from build123d import *

# Parameters (mm, degrees)
SKETCH1_R           = 48.895
SKETCH1_R_2         = 45.72
BOSS_EXTRUDE1_DEPTH = 6.35
SKETCH2_R           = 48.895
SKETCH2_R_2         = 12.7
BOSS_EXTRUDE2_DEPTH = 3.175
SKETCH3_R           = 3.175
BOSS_EXTRUDE3_DEPTH = 46.825


with BuildPart() as part:
    # Sketch1 → Boss-Extrude1 (new body)
    with BuildSketch(Plane(origin=(0, 0, 0), x_dir=(1, 0, 0), z_dir=(0, 1, 0))):
        with Locations(Location((0, 0, 0), (0, 0, 270))):
            Circle(SKETCH1_R)
        with Locations(Location((0, 0, 0), (0, 0, 270))):
            Circle(SKETCH1_R_2, mode=Mode.SUBTRACT)
    extrude(amount=BOSS_EXTRUDE1_DEPTH)

    # Sketch2 → Boss-Extrude2 (add)
    with BuildSketch(Plane(origin=(0, 6.35, 0), x_dir=(1, 0, 0), z_dir=(0, 1, 0))):
        with Locations(Location((0, 0, 0), (0, 0, 270))):
            Circle(SKETCH2_R)
        with Locations(Location((0, 25.4, 0), (0, 0, 270))):
            Circle(SKETCH2_R_2, mode=Mode.SUBTRACT)
        with Locations(Location((25.4, 0, 0), (0, 0, 270))):
            Circle(SKETCH2_R_2, mode=Mode.SUBTRACT)
        with Locations(Location((0, -25.4, 0), (0, 0, 270))):
            Circle(SKETCH2_R_2, mode=Mode.SUBTRACT)
        with Locations(Location((-25.4, 0, 0), (0, 0, 270))):
            Circle(SKETCH2_R_2, mode=Mode.SUBTRACT)
    extrude(amount=BOSS_EXTRUDE2_DEPTH)

    # Sketch3 → Boss-Extrude3 (add)
    with BuildSketch(Plane(origin=(0, 9.525, 0), x_dir=(1, 0, 0), z_dir=(0, 1, 0))):
        with Locations(Location((0, 0, 0), (0, 0, 270))):
            Circle(SKETCH3_R)
    extrude(amount=BOSS_EXTRUDE3_DEPTH)


solid = part.part
Design review of the part built by this model. Coordinates are the model's own, in mm. A direction names the side the tool comes from. Coordinates: 2 decimals unless noted, no trailing zeros. Loops run counter-clockwise (first coordinate to the right, second up) from the corner with the lowest first, then second, coordinate; pieces in that order, holes last. Notation, with made-up numbers: M 15,20.25 L 20,20.25 A12 cw 20,41.25 Z; hole C 52,-13.5 d7. An arc over 180 degrees is marked long. Answer as CSV lines item,"result".
Item 1: Add section B-B on x = -5.5. State the section outline as (y, z) points (3 decimals), plus the area to 3 significant figures.
Answer list:
outline,"M 0,-48.585 L 9.525,-48.585 L 9.525,-36.847 L 6.35,-36.847 L 6.35,-45.388 L 0,-45.388 Z; M 0,45.388 L 6.35,45.388 L 6.35,36.847 L 9.525,36.847 L 9.525,48.585 L 0,48.585 Z; M 6.35,-13.953 L 9.525,-13.953 L 9.525,13.953 L 6.35,13.953 Z"
area,"204 mm²"
Item 2: For probe 1 along X at (y, z) = (7.1, 0) (3 decimals); probe 2 along X at (y, z) = (4, 0) (3 decimals); probe 3 along Y at (x, z) = (29.5, -37) (3 decimals), list the stretches that pass through material, from the lowest coordinate up.
Answer list:
probe 1,"-48.895 to -38.1, -12.7 to 12.7, 38.1 to 48.895"
probe 2,"-48.895 to -45.72, 45.72 to 48.895"
probe 3,"0 to 9.525"
Item 3: Add section D-D on x = 25.4. State the section outline as (y, z) points (3 decimals), plus the area to 3 significant figures.
Answer list:
outline,"M 0,-41.78 L 9.525,-41.78 L 9.525,-12.7 L 6.35,-12.7 L 6.35,-38.015 L 0,-38.015 Z; M 0,38.015 L 6.35,38.015 L 6.35,12.7 L 9.525,12.7 L 9.525,41.78 L 0,41.78 Z"
area,"232 mm²"
Item 4: Add section A-A on z = 0. State the section outline as (x, y) points (3 decimals), plus the area to 3 significant figures.
Answer list:
outline,"M -48.895,0 L -45.72,0 L -45.72,6.35 L -38.1,6.35 L -38.1,9.525 L -48.895,9.525 Z; M -12.7,6.35 L 12.7,6.35 L 12.7,9.525 L 3.175,9.525 L 3.175,56.35 L -3.175,56.35 L -3.175,9.525 L -12.7,9.525 Z; M 38.1,6.35 L 45.72,6.35 L 45.72,0 L 48.895,0 L 48.895,9.525 L 38.1,9.525 Z"
area,"487 mm²"
Item 5: For P1, Ø8, axis at x = 27.5, z = 26, coming from the +Y side (3 decimals); P2, Ø1, axis at y = 9.5, z = -7, coming from the +X side; P3, Ø8, axis at y = 9.5, z = 4.5, coming from the +X side, all flat-tipped, find the tip position at first contact; note any pin that passes through.
Answer list:
P1,"y = 9.525"
P2,"x = 48.46"
P3,"x = 48.89"
Item 6: The part is to be moulded in two halves that separate along Z. For faces 1 (the face through (-37.8, 7.92, -2.75)), 2 (the face through (-36, 0, 29)), 3 (the face through (-47.732, 4.696, -10.599)), say which applies: pulls with the +Z half, pulls with the -Z half, needs draft (parallel to the pull), parting line crosses it, or undercut.
Answer list:
face 1,"undercut"
face 2,"needs draft"
face 3,"parting line crosses it"
Item 7: Add section C-C on z = -20.5. State the section outline as (x, y) points (3 decimals), plus the area to 3 significant figures.
Answer list:
outline,"M -44.39,0 L -40.866,0 L -40.866,6.35 L -11.717,6.35 L -11.717,9.525 L -44.39,9.525 Z; M 11.717,6.35 L 40.866,6.35 L 40.866,0 L 44.39,0 L 44.39,9.525 L 11.717,9.525 Z"
area,"252 mm²"
Item 8: Machinability: for faces 4 (the face through (37.992, 7.915, -1.653)), 5 (the face through (-1.93, 32.61, -2.52)), 6 (the face through (1, 6.35, -1)), which of the approach directions +Z, -Z, +X, -X, +Y, -Y give a long, thin tool a straight path to every point of the face, cutting with its end or side? Answer none if there is none.
Answer list:
face 4,"+Y, -Y"
face 5,"+Y"
face 6,"-Y"
